Build history of the part. All positions in model axes, mm. Give positions to 0.01 mm unless a question says otherwise; leave off trailing zeros. Loops run counter-clockwise (first coordinate to the right, second up) from the corner with the lowest first, then second, coordinate; pieces in that order, holes last. Notation, with made-up numbers: (82, 10) -> (110, 10) arc R21 cw to (110, 49) -> close; hole circle Ø6 at (-12.5, 89). An arc over 180 degrees is marked (long way). One line per question, with ' | ' between items. Start each with the question number.
(1) Slice it at B-B, the plane z = 102. Write the cut outline in (x, y).
(2) Drill centre lines: L1, parallel to Y at x = -5, z = 447; L2, parallel to Y at x = -6, z = 52; L3, parallel to Y at x = 2, z = 322.5. Where is each one in solid material? Low to high. Write a range as from..to.
(3) Flat gauge pins, fed straight in: pin 1 Ø4 at (x, z) = (1.5, 798) entering from +Y; pin 2 Ø10 at (y, z) = (7, 706) entering from -X; pin 3 Ø1.5 at (y, z) = (14.5, 640) entering from -X. Where does each tip first touch, or does it go through?
(4) Slice it at A-A, the plane y = 7. Give the number of separate pieces and of enclosed holes in the cut face, then the cut area to 3 significant figures.
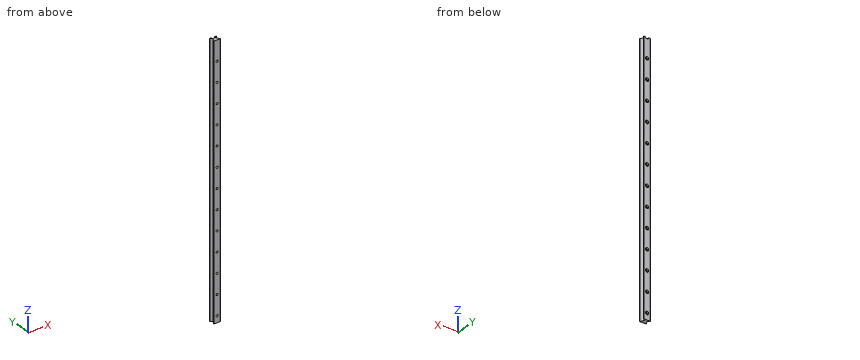
```python
from build123d import *

# Parameters (mm, degrees)
PAD_DEPTH       = 800
SKETCH001_R     = 3
POCKET_DEPTH    = 17.410023
SKETCH002_R     = 5
POCKET001_DEPTH = 5


with BuildPart() as part:
    # Sketch → Pad (new body)
    with BuildSketch(Plane.XY):
        with BuildLine():
            Line((-9.5, 0), (9.5, 0))
            ThreePointArc((9.5, 0), (9.928584, 0.242481), (9.941474, 0.734736))
            Line((4, 11.909023), (9.941474, 0.734736))
            Line((9.810688, 16.517266), (4, 11.909023))
            ThreePointArc((9.810688, 16.517266), (9.972164, 17.073525), (9.5, 17.409023))
            Line((9.5, 17.409023), (-9.5, 17.409023))
            ThreePointArc((-9.5, 17.409023), (-9.972164, 17.073525), (-9.810688, 16.517266))
            Line((-9.810688, 16.517266), (-4, 11.909023))
            Line((-4, 11.909023), (-9.941474, 0.734736))
            ThreePointArc((-9.941474, 0.734736), (-9.928584, 0.242481), (-9.5, 0))
        make_face()
    extrude(amount=PAD_DEPTH)

    # Sketch001 (on Face2 of Pad) → Pocket (cut, through all)
    with BuildSketch(Plane(origin=(0, 17.409023, 0), x_dir=(-1, 0, 0), z_dir=(0, 1, 0))):
        with Locations((0, 20)):
            Circle(SKETCH001_R)
        with Locations((0, 80)):
            Circle(SKETCH001_R)
        with Locations((0, 140)):
            Circle(SKETCH001_R)
        with Locations((0, 200)):
            Circle(SKETCH001_R)
        with Locations((0, 260)):
            Circle(SKETCH001_R)
        with Locations((0, 320)):
            Circle(SKETCH001_R)
        with Locations((0, 380)):
            Circle(SKETCH001_R)
        with Locations((0, 440)):
            Circle(SKETCH001_R)
        with Locations((0, 500)):
            Circle(SKETCH001_R)
        with Locations((0, 560)):
            Circle(SKETCH001_R)
        with Locations((0, 620)):
            Circle(SKETCH001_R)
        with Locations((0, 680)):
            Circle(SKETCH001_R)
        with Locations((0, 740)):
            Circle(SKETCH001_R)
    extrude(amount=-POCKET_DEPTH, mode=Mode.SUBTRACT)

    # Sketch002 (on Face3 of Pocket) → Pocket001 (cut)
    with BuildSketch(Plane(origin=(0, 17.409023, 0), x_dir=(-1, 0, 0), z_dir=(0, 1, 0))):
        with Locations((0, 20)):
            Circle(SKETCH002_R)
        with Locations((0, 80)):
            Circle(SKETCH002_R)
        with Locations((0, 140)):
            Circle(SKETCH002_R)
        with Locations((0, 200)):
            Circle(SKETCH002_R)
        with Locations((0, 260)):
            Circle(SKETCH002_R)
        with Locations((0, 320)):
            Circle(SKETCH002_R)
        with Locations((0, 380)):
            Circle(SKETCH002_R)
        with Locations((0, 440)):
            Circle(SKETCH002_R)
        with Locations((0, 500)):
            Circle(SKETCH002_R)
        with Locations((0, 560)):
            Circle(SKETCH002_R)
        with Locations((0, 620)):
            Circle(SKETCH002_R)
        with Locations((0, 680)):
            Circle(SKETCH002_R)
        with Locations((0, 740)):
            Circle(SKETCH002_R)
        with Locations((0, 800)):
            Circle(SKETCH002_R)
    extrude(amount=-POCKET001_DEPTH, mode=Mode.SUBTRACT)


solid = part.part
```
Final values:
1) outline: (-9.94, 0.73) arc R0.5 ccw to (-9.5, 0) -> (9.5, 0) arc R0.5 ccw to (9.94, 0.73) -> (4, 11.91) -> (9.81, 16.52) arc R0.5 ccw to (9.5, 17.41) -> (-9.5, 17.41) arc R0.5 ccw to (-9.81, 16.52) -> (-4, 11.91) -> close
2) L1: 0..10.03, 12.7..17.41 | L2: 0..8.15, 13.5..17.41 | L3: 0..12.41
3) pin 1: y = 12.41 | pin 2: x = -9.27 | pin 3: x = -8.21
4) separate pieces: 1 | enclosed holes: 13 | area: 10,200 mm2
